```python
from build123d import *

# Parameters (mm, degrees)
SKETCH023_W     = 69
SKETCH023_H     = 88
SKETCH023_R     = 1.3
PAD006_DEPTH    = 14
SKETCH024_W     = 59
SKETCH024_H     = 78
POCKET014_DEPTH = 11
SKETCH025_R     = 3
SKETCH025_R_2   = 2.5
POCKET015_DEPTH = 1
FILLET006_R     = 7
FILLET007_R     = 2
SKETCH026_W     = 14
SKETCH026_H     = 8.5
POCKET016_DEPTH = 10


with BuildPart() as part:
    # Sketch023 → Pad006 (new body)
    with BuildSketch(Plane.XY):
        with Locations((34.5, 44)):
            Rectangle(SKETCH023_W, SKETCH023_H)
        with Locations((15.5, 63)):
            Circle(SKETCH023_R, mode=Mode.SUBTRACT)
        with Locations((15.5, 44)):
            Circle(SKETCH023_R, mode=Mode.SUBTRACT)
        with Locations((15.5, 25)):
            Circle(SKETCH023_R, mode=Mode.SUBTRACT)
        with Locations((53.5, 25)):
            Circle(SKETCH023_R, mode=Mode.SUBTRACT)
        with Locations((53.5, 44)):
            Circle(SKETCH023_R, mode=Mode.SUBTRACT)
        with Locations((53.5, 63)):
            Circle(SKETCH023_R, mode=Mode.SUBTRACT)
    extrude(amount=PAD006_DEPTH)

    # Sketch024 (on Face12 of Pad006) → Pocket014 (cut)
    with BuildSketch(Plane.XY.offset(14)):
        with Locations((34.5, 44)):
            Rectangle(SKETCH024_W, SKETCH024_H)
    extrude(amount=-POCKET014_DEPTH, mode=Mode.SUBTRACT)

    # Sketch025 (on Face4 of Pocket014) → Pocket015 (cut)
    with BuildSketch(Plane(origin=(0, 0, 0), x_dir=(1, 0, 0), z_dir=(0, 0, -1))):
        with Locations((6, -6)):
            Circle(SKETCH025_R)
        with Locations((63, -6)):
            Circle(SKETCH025_R)
        with Locations((63, -82)):
            Circle(SKETCH025_R)
        with Locations((6, -82)):
            Circle(SKETCH025_R)
        with Locations((15.5, -25)):
            Circle(SKETCH025_R_2)
        with Locations((15.5, -44)):
            Circle(SKETCH025_R_2)
        with Locations((15.5, -63)):
            Circle(SKETCH025_R_2)
        with Locations((53.5, -63)):
            Circle(SKETCH025_R_2)
        with Locations((53.5, -44)):
            Circle(SKETCH025_R_2)
        with Locations((53.5, -25)):
            Circle(SKETCH025_R_2)
    extrude(amount=-POCKET015_DEPTH, mode=Mode.SUBTRACT)

    # Fillet006
    fillet006_edges = [part.edges().sort_by_distance(p)[0] for p in [
        (69, 88, 7),
        (0, 88, 7),
        (0, 0, 7),
        (69, 0, 7),
    ]]
    fillet(fillet006_edges, radius=FILLET006_R)

    # Fillet007
    fillet007_edges = [part.edges().sort_by_distance(p)[0] for p in [
        (64, 5, 8.5),
        (64, 83, 8.5),
        (5, 83, 8.5),
        (5, 5, 8.5),
        (0, 44, 14),
        (0, 44, 0),
    ]]
    fillet(fillet007_edges, radius=FILLET007_R)

    # Sketch026 (on Face13 of Fillet007) → Pocket016 (cut)
    with BuildSketch(Plane.YZ.offset(69)):
        with Locations((53.5, 6.75)):
            Rectangle(SKETCH026_W, SKETCH026_H)
    extrude(amount=-POCKET016_DEPTH, mode=Mode.SUBTRACT)


solid = part.part
```
Here's how the part is built. I have some questions about the finished solid (model axes, mm). A direction names the side the tool comes from. Round coordinates to 2 decimals unless told otherwise and drop trailing zeros. Order: outer loops, then holes, each group sorted by start corner. A loop starts at its lowest first (then second) coordinate and runs counter-clockwise, first axis right, second up. Notation, with made-up numbers: M 48.25,-29 L 71.25,-29 A23 ccw 71.25,-5 Z; hole C 12.25,65.25 d6. An arc over 180 degrees is marked long. Use CSV: the item, a comma, the result in double quotes.
1) I want a section at A-A (y = 44). List the corners of the cut face in (x, z) for me.
Taken from the geometry:
outline,"M 0,2 A2 ccw 2,0 L 13,0 L 13,1 L 14.2,1 L 14.2,3 L 5,3 L 5,14 L 2,14 A2 ccw 0,12 Z; M 16.8,1 L 18,1 L 18,0 L 51,0 L 51,1 L 52.2,1 L 52.2,3 L 16.8,3 Z; M 54.8,1 L 56,1 L 56,0 L 67,0 A2 ccw 69,2 L 69,12 A2 ccw 67,14 L 64,14 L 64,3 L 54.8,3 Z"
2) On a 3-axis mill with a long thin cutter (end or side, diameter ignored), from which of +Z, -Z, +X, -X, +Y, -Y can I reach the whole of each face in a straight line? I mean faces 1 (the cylindrical face through (34.11, 0.57, 13.4)), 2 (the cylindrical face through (5.6, 82.43, 8.42)), 3 (the flat face through (55, 45, 1)). Say none if no direction works.
Taken from the geometry:
face 1,"+Z, +X, -X, -Y"
face 2,"+Z"
face 3,"-Z"
3) I need wall thicknesses on line 1 along Y through (x, z) = (15.5, 2.1); line 2 along X through (y, z) = (25, 2.2); line 3 along X through (y, z) = (8, 11). Which ranges of each line are inside material? Lowest first, please. Write a range as [from, to].
Taken from the geometry:
line 1,"[0, 23.7], [26.3, 42.7], [45.3, 61.7], [64.3, 88]"
line 2,"[0, 14.2], [16.8, 52.2], [54.8, 69]"
line 3,"[0, 5], [64, 69]"
4) I want a section at C-C (z = 5.5). List the corners of the cut face in (x, y) for me, then the cut area to 3 significant figures.
Taken from the geometry:
outline,"M 0,7 A7 ccw 7,0 L 62,0 A7 ccw 69,7 L 69,46.5 L 64,46.5 L 64,7 A2 cw 62,5 L 7,5 A2 cw 5,7 L 5,81 A2 cw 7,83 L 62,83 A2 cw 64,81 L 64,60.5 L 69,60.5 L 69,81 A7 ccw 62,88 L 7,88 A7 ccw 0,81 Z"
area,"1,360 mm^2"
5) I want a section at D-D (y = 17). List the corners of the cut face in (x, z) for me.
Taken from the geometry:
outline,"M 0,2 A2 ccw 2,0 L 67,0 A2 ccw 69,2 L 69,12 A2 ccw 67,14 L 64,14 L 64,3 L 5,3 L 5,14 L 2,14 A2 ccw 0,12 Z"
6) I want a section at B-B (x = 53.5). Count the separate pieces of the cut face and the enclosed holes in it, then the cut area to 3 significant figures.
Taken from the geometry:
separate pieces,"4"
enclosed holes,"0"
area,"340 mm^2"
7) I'm going to push flat-ended pins straight in: P1, Ø3, axis at x = 19, y = 38.5, coming from the +Z side; P2, Ø5.5, axis at x = 6, y = 82, coming from the -Z side. Where does each tip first touch, or does it pass through?
Taken from the geometry:
P1,"z = 3"
P2,"z = 1"
8) If we mould it in two halves opening along X, with no side actions, what happens to faces 4 (the cylindrical face through (34.89, 87.43, 13.4)), 5 (the cylindrical face through (54.84, 22.89, 0.49)), 6 (the cylindrical face through (2, 85.9, 7.1))? For each: pulls with the +X half, pulls with the -X half, needs draft (parallel to the pull), parting line crosses it, or undercut.
Taken from the geometry:
face 4,"needs draft"
face 5,"undercut"
face 6,"pulls with the -X half"
